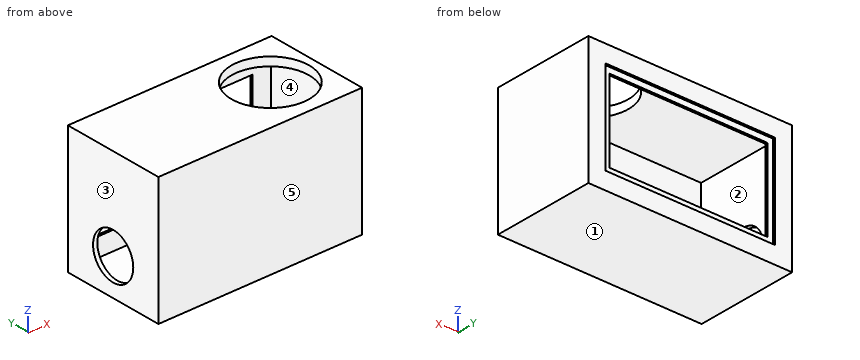
```python
from build123d import *

# Parameters (mm, degrees)
F0_W      = 901.7
F0_H      = 527.05
F1_DEPTH  = 457.2
F2_T      = -19.05
F3_W      = 901.7
F3_H      = 457.2
F4_DEPTH  = 38.1
F5_R      = 101.6
F6_DEPTH  = 19.05
F7_R      = 171.45
F8_DEPTH  = 38.1
F9_W      = 749.3
F9_H      = 412.75
F10_DEPTH = 9.525
F11_W     = 698.5
F11_H     = 361.95
F12_DEPTH = 9.525


with BuildPart() as f1:
    # F0 (on Front) → F1 (new body)
    with BuildSketch(Plane.XZ):
        Rectangle(F0_W, F0_H)
    extrude(amount=F1_DEPTH)

    # F2
    f2_openings = [f1.faces().sort_by_distance(p)[0] for p in [
        (0, -228.6, 263.525),
    ]]
    offset(amount=F2_T, openings=f2_openings)

    # F3 (on face) → F4 (join)
    with BuildSketch(Plane.XY.offset(263.525)):
        with Locations((0, -228.6)):
            Rectangle(F3_W, F3_H)
    extrude(amount=F4_DEPTH)

    # F5 (on face) → F6 (cut, through all)
    with BuildSketch(Plane(origin=(-450.85, 0, 0), x_dir=(0, -1, 0), z_dir=(-1, 0, 0))):
        with Locations((228.6, -102.11508)):
            Circle(F5_R)
    extrude(amount=-F6_DEPTH, mode=Mode.SUBTRACT)

    # F7 (on face) → F8 (cut, through all)
    with BuildSketch(Plane.XY.offset(301.625)):
        with Locations((244.839686, -228.6)):
            Circle(F7_R)
    extrude(amount=-F8_DEPTH, mode=Mode.SUBTRACT)

    # F9 (on face) → F10 (cut)
    with BuildSketch(Plane(origin=(0, 0, 0), x_dir=(-1, 0, 0), z_dir=(0, 1, 0))):
        with Locations((0, 19.05)):
            Rectangle(F9_W, F9_H)
    extrude(amount=-F10_DEPTH, mode=Mode.SUBTRACT)

    # F11 (on face) → F12 (cut, through all)
    with BuildSketch(Plane(origin=(0, -9.525, 0), x_dir=(-1, 0, 0), z_dir=(0, 1, 0))):
        with Locations((0, 19.05)):
            Rectangle(F11_W, F11_H)
    extrude(amount=-F12_DEPTH, mode=Mode.SUBTRACT)


solid = f1.part
```
The model under review builds one solid part; all positions refer to its coordinate system, in mm. Face numbers are marked on the shaded views. A direction names the side the tool comes from. Give positions to 0.01 mm unless a question says otherwise; leave off trailing zeros. Write each loop counter-clockwise with the first axis right and the second up, starting at its lowest first coordinate (ties: lowest second). Pieces come first, ordered by that corner, then holes. Notation, with made-up numbers: M -32.5,64 L -13.5,64 A24 ccw -13.5,74 Z; hole C -1.75,-5.5 d10. An arc over 180 degrees is marked long. Write each question's results on one line, items separated by ' | '. Start each with the question number.
1. Insertion check: pin 1 Ø1 at (x, z) = (199, 179) entering from +Y. The pin has a flat end and moves straight along its axis. Give the tip position at first contact, or say it passes through.
2. For the marked faces 4 and 5, list the 3-axis set-ups (+Z, -Z, +X, -X, +Y, -Y) from which the entire face can be reached by the end or side of a thin tool; tool diameter is ignored.
3. Mouldability with a two-part tool opening along X and no side actions: class the marked faces 1, 2 and 3 as released by +X, released by -X, zero draft, split by the parting line, or undercut.
4. We need section B-B (y = -228.6). Write out the cut boundary in (x, z) (3 decimals), and give its area (3 significant figures).
5. For probe 1 along Y at (x, z) = (265, 200.5) (3 decimals); probe 2 along Y at (x, z) = (-205, 243.5); probe 3 along Z at (x, y) = (-447, -228.6) (3 decimals), list the stretches that pass through material, from the lowest coordinate up. Write a range as [from, to].
6. We need section D-D (y = -45.5). Write out the cut boundary in (x, z) (3 decimals), and give its area (3 significant figures).
7. We need section A-A (z = 242). Write out the cut boundary in (x, y).
8. We need section C-C (x = 179). Write out the cut boundary in (y, z) (3 decimals).
Results found:
1) pin 1: stops at y = -438.15
2) face 4: none | face 5: +Z, -Z, +X, -X, -Y
3) face 1: zero draft | face 2: undercut | face 3: released by -X
4) outline: M -450.85,-263.525 L 450.85,-263.525 L 450.85,301.625 L 416.29,301.625 L 416.29,263.525 L 431.8,263.525 L 431.8,-244.475 L -431.8,-244.475 L -431.8,-203.715 L -450.85,-203.715 Z; M -450.85,-0.515 L -431.8,-0.515 L -431.8,263.525 L 73.39,263.525 L 73.39,301.625 L -450.85,301.625 Z | area: 54,000 mm^2
5) probe 1: y = [-457.2, -438.15], [-19.05, -9.525] | probe 2: y = [-457.2, -438.15], [-19.05, 0] | probe 3: z = [-263.525, -203.715], [-0.515, 301.625]
6) outline: M -450.85,-263.525 L 450.85,-263.525 L 450.85,301.625 L -450.85,301.625 Z; hole M -431.8,-244.475 L 431.8,-244.475 L 431.8,263.525 L -431.8,263.525 Z | area: 70,900 mm^2
7) outline: M -450.85,-457.2 L 450.85,-457.2 L 450.85,0 L -450.85,0 Z; hole M -431.8,-438.15 L 431.8,-438.15 L 431.8,-19.05 L -431.8,-19.05 Z
8) outline: M -457.2,-263.525 L 0,-263.525 L 0,-187.325 L -9.525,-187.325 L -9.525,-161.925 L -19.05,-161.925 L -19.05,-244.475 L -438.15,-244.475 L -438.15,263.525 L -386.904,263.525 L -386.904,301.625 L -457.2,301.625 Z; M -70.296,263.525 L -19.05,263.525 L -19.05,200.025 L -9.525,200.025 L -9.525,225.425 L 0,225.425 L 0,301.625 L -70.296,301.625 Z
